from build123d import *

# Parameters (mm, degrees)
F0_W     = 33.401
F0_H     = 33.401
F0_R     = 15.113
F1_DEPTH = 19.9644
F2_R     = 16.70049
F3_R     = 0.79375


# Not quite as in the source:
# - a fillet or chamfer is up to 0.001 mm smaller than in the source, because OpenCascade refuses the exact size


with BuildPart() as f1:
    # F0 (on Top) → F1 (new body)
    with BuildSketch(Plane.XY):
        Rectangle(F0_W, F0_H)
        Circle(F0_R, mode=Mode.SUBTRACT)
    extrude(amount=F1_DEPTH)

    # F2 (radius 16.7005 in the source; OpenCascade refuses exactly that, so slightly less here)
    f2_edges = [f1.edges().sort_by_distance(p)[0] for p in [
        (-16.7005, -16.7005, 9.9822),
        (16.7005, -16.7005, 9.9822),
    ]]
    fillet(f2_edges, radius=F2_R)

    # F3
    f3_edges = [f1.edges().sort_by_distance(p)[0] for p in [
        (11.80904, -11.80904, 19.9644),
        (11.80904, -11.80904, 0),
    ]]
    fillet(f3_edges, radius=F3_R)


solid = f1.part
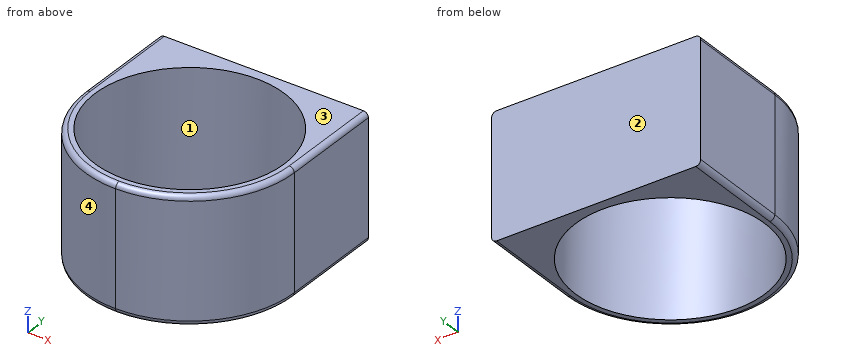
Build history of the part. All positions in model axes, mm. Face numbers are marked on the shaded views. Round coordinates to 2 decimals unless told otherwise and drop trailing zeros. Write each loop counter-clockwise with the first axis right and the second up, starting at its lowest first coordinate (ties: lowest second). Pieces come first, ordered by that corner, then holes. Notation, with made-up numbers: M -1,78.5 L 40,78.5 A28 cw 40,107.5 Z; hole C 11.25,83 d5. An arc over 180 degrees is marked long. Answer as a JSON object with one key per item and string values. Group by question number.
(1) Flat gauge pins, fed straight in: pin 1 (4 mm diameter, centred on x = 10.5, z = 10, fed in from -Y); pin 2 (4 mm diameter, centred on x = 1, y = -11.5, fed in from +Z); pin 3 (3 mm diameter, centred on x = -5, z = 5, fed in from -Y). Where does each tip first touch, or does it go through?
(2) Drill centre lines: L1, parallel to Y at x = 0, z = 14.5; L2, parallel to X at y = -7, z = 6; L3, parallel to X at y = 12, z = 3.75. Where is each one in solid material? Low to high.
(3) Cut at B-B (y = 9.5). Give the cut face in (x, z).
(4) Cut at C-C (y = 6). Give the cut face in (x, z).
(5) Mould opens along Y. For the marked faces 1, 2, 3 and 4 say: pulls with the +Y half, pulls with the -Y half, needs draft (parallel to the pull), parting line crosses it, or undercut.
Responses:
{
 "1": {"pin 1": "stops at y = -14.38", "pin 2": "passes through", "pin 3": "stops at y = -16.33"},
 "2": {"L1": "y = -16.7 to -15.11, 15.11 to 16.7", "L2": "x = -15.16 to -13.39, 13.39 to 15.16", "L3": "x = -16.7 to -9.19, 9.19 to 16.7"},
 "3": {"outline": "M -16.7,0.79 A0.79 ccw -15.91,0 L -11.75,0 L -11.75,19.96 L -15.91,19.96 A0.79 ccw -16.7,19.17 Z; M 11.75,0 L 15.91,0 A0.79 ccw 16.7,0.79 L 16.7,19.17 A0.79 ccw 15.91,19.96 L 11.75,19.96 Z"},
 "4": {"outline": "M -16.7,0.79 A0.79 ccw -15.91,0 L -13.87,0 L -13.87,19.96 L -15.91,19.96 A0.79 ccw -16.7,19.17 Z; M 13.87,0 L 15.91,0 A0.79 ccw 16.7,0.79 L 16.7,19.17 A0.79 ccw 15.91,19.96 L 13.87,19.96 Z"},
 "5": {"face 1": "undercut", "face 2": "pulls with the +Y half", "face 3": "needs draft", "face 4": "pulls with the -Y half"}
}
